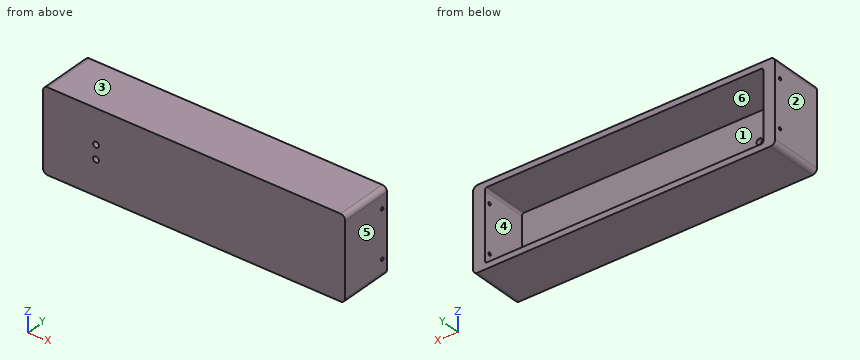
from build123d import *

# Parameters (mm, degrees)
SKETCH1_W           = 326.39
SKETCH1_H           = 88.9
SKETCH1_W_2         = 300.99
SKETCH1_H_2         = 76.2
BOSS_EXTRUDE1_DEPTH = 50.8
SKETCH2_W           = 326.39
SKETCH2_H           = 88.9
BOSS_EXTRUDE2_DEPTH = 6.35
SKETCH3_R           = 3.1
CUT_EXTRUDE1_DEPTH  = 179.534402917
SKETCH4_R           = 1.6875
CUT_EXTRUDE3_DEPTH  = 313.69
FILLET1_R           = 5.08
FILLET2_R           = 2.54


with BuildPart() as part:
    # Sketch1 → Boss-Extrude1 (new body)
    with BuildSketch(Plane(origin=(0, 0, 0), x_dir=(1, 0, 0), z_dir=(0, 1, 0))):
        Rectangle(SKETCH1_W, SKETCH1_H)
        Rectangle(SKETCH1_W_2, SKETCH1_H_2, mode=Mode.SUBTRACT)
    extrude(amount=BOSS_EXTRUDE1_DEPTH)

    # Sketch2 → Boss-Extrude2 (add)
    with BuildSketch(Plane.XZ):
        Rectangle(SKETCH2_W, SKETCH2_H)
    extrude(amount=BOSS_EXTRUDE2_DEPTH)

    # Sketch3 → Cut-Extrude1 (cut, through all)
    with BuildSketch(Plane.XZ.offset(6.35)):
        with Locations(Location((-106, 7.5, 0), (0, 0, 270))):
            Circle(SKETCH3_R)
        with Locations(Location((-106, -7.5, 0), (0, 0, 270))):
            Circle(SKETCH3_R)
    extrude(amount=-CUT_EXTRUDE1_DEPTH, mode=Mode.SUBTRACT)

    # Sketch4 → Cut-Extrude3 (cut)
    with BuildSketch(Plane(origin=(163.195, 0, 0), x_dir=(0, 0, -1), z_dir=(1, 0, 0))):
        with Locations((25.4, 44.22394)):
            Circle(SKETCH4_R)
        with Locations(Location((-25.4, 44.22394, 0), (0, 0, 180))):
            Circle(SKETCH4_R)
    cut_extrude3 = extrude(amount=-CUT_EXTRUDE3_DEPTH, mode=Mode.SUBTRACT)

    # Mirror2: Cut-Extrude3 across plane
    add(cut_extrude3.mirror(Plane(origin=(0, 0, 0), x_dir=(0, 0, 1), z_dir=(1, 0, 0))), mode=Mode.SUBTRACT)

    # Fillet1
    fillet1_edges = [part.edges().sort_by_distance(p)[0] for p in [
        (163.195, 22.225, 44.45),
        (-163.195, 22.225, 44.45),
        (-163.195, 22.225, -44.45),
        (163.195, 22.225, -44.45),
    ]]
    fillet(fillet1_edges, radius=FILLET1_R)

    # Fillet2
    fillet2_edges = [part.edges().sort_by_distance(p)[0] for p in [
        (150.495, 25.4, 38.1),
        (150.495, 25.4, -38.1),
        (-150.495, 25.4, -38.1),
        (-150.495, 25.4, 38.1),
    ]]
    fillet(fillet2_edges, radius=FILLET2_R)


solid = part.part
Input: part model. Units: mm. Frame: model coordinates. Face numbers are marked on the shaded views. A direction names the side the tool comes from. Coordinates: 2 decimals unless noted, no trailing zeros. Loops run counter-clockwise (first coordinate to the right, second up) from the corner with the lowest first, then second, coordinate; pieces in that order, holes last. Notation, with made-up numbers: (73.25, -5) -> (123.25, -5) arc R17 cw to (123.25, 25) -> close; hole circle Ø5 at (5.25, -28). An arc over 180 degrees is marked (long way). One line per item, written item: value.
(1) Cut plane C-C (x = -106). Output: boundary loops of the cut face in (y, z), then the cut area to 3 significant figures.
Answer below:
outline: (-6.35, -44.45) -> (50.8, -44.45) -> (50.8, -38.1) -> (0, -38.1) -> (0, -10.6) -> (-6.35, -10.6) -> close; (-6.35, -4.4) -> (0, -4.4) -> (0, 4.4) -> (-6.35, 4.4) -> close; (-6.35, 10.6) -> (0, 10.6) -> (0, 38.1) -> (50.8, 38.1) -> (50.8, 44.45) -> (-6.35, 44.45) -> close
area: 1,130 mm2
(2) Ray query, line 1 along X through (y, z) = (22.5, -21) (3 decimals); line 2 along Z through (x, y) = (146.5, 6.5); line 3 along X through (y, z) = (-5, 7) (3 decimals). Return the intervals inside material, ascending.
Answer below:
line 1: x = -163.195 to -150.495, 150.495 to 163.195
line 2: z = -44.45 to -38.1, 38.1 to 44.45
line 3: x = -163.195 to -109.059, -102.941 to 163.195
(3) Cut plane A-A (x = -56). Output: boundary loops of the cut face in (y, z).
Answer below:
outline: (-6.35, -44.45) -> (50.8, -44.45) -> (50.8, -38.1) -> (0, -38.1) -> (0, 38.1) -> (50.8, 38.1) -> (50.8, 44.45) -> (-6.35, 44.45) -> close
(4) Cut plane D-D (z = 31.5). Output: boundary loops of the cut face in (x, y) (3 decimals), then the cut area to 3 significant figures.
Answer below:
outline: (-163.195, -6.35) -> (163.195, -6.35) -> (163.195, 50.8) -> (150.495, 50.8) -> (150.495, 0) -> (-150.495, 0) -> (-150.495, 50.8) -> (-163.195, 50.8) -> close
area: 3,360 mm2
(5) Set-up query: the marked faces 1 and 2. Return all of +Z, -Z, +X, -X, +Y, -Y with unobstructed straight access to the full face (end or side cutting, diameter ignored); none if empty.
Answer below:
face 1: +Y
face 2: +Z, -Z, -X, +Y, -Y
(6) Pin query (flat end, axial travel): pin 1 Ø8 at (x, z) = (-106, 7.5) entering from +Y. Return the tip coordinate at first contact, or that it passes through.
Answer below:
pin 1: stops at y = 0
(7) Cut plane B-B (z = -7.5). Output: boundary loops of the cut face in (x, y) (3 decimals), then the cut area to 3 significant figures.
Answer below:
outline: (-163.195, -6.35) -> (-109.1, -6.35) -> (-109.1, 0) -> (-150.495, 0) -> (-150.495, 50.8) -> (-163.195, 50.8) -> close; (-102.9, -6.35) -> (163.195, -6.35) -> (163.195, 50.8) -> (150.495, 50.8) -> (150.495, 0) -> (-102.9, 0) -> close
area: 3,320 mm2
(8) Draft query along Z for the marked faces 3, 4, 5 and 6. Return one class per face: pulls with the +Z half, pulls with the -Z half, needs draft (parallel to the pull), parting line crosses it, or undercut.
Answer below:
face 3: pulls with the +Z half
face 4: undercut
face 5: needs draft
face 6: undercut
